CAD build for the part. Positions are in the model's coordinates, mm. Face numbers are marked on the shaded views. Coordinates: 2 decimals unless noted, no trailing zeros. Order: outer loops, then holes, each group sorted by start corner. A loop starts at its lowest first (then second) coordinate and runs counter-clockwise, first axis right, second up. Notation, with made-up numbers: M -9.75,-10.5 L 46.25,-10.5 A30 ccw 46.25,20.5 Z; hole C 74,-32.5 d10. An arc over 180 degrees is marked long. Write item = value, one per line.
from build123d import *


with BuildPart() as f1:
    # F0 (on Front) → F1 (revolve)
    with BuildSketch(Plane.XZ):
        Polygon((-22, 0), (-17, 0), (-16.25, 45), (-20.25, 45), align=None)
    revolve(axis=Axis((0, 0, 22.5), (0, 0, 1)))

    # F0 (on Front) → F2 (revolve)
    with BuildSketch(Plane.XZ):
        with BuildLine():
            Line((-20.25, 45), (-16.25, 45))
            Line((-16.25, 45), (-10.1249999976, 59.999902775))
            add(Edge.make_bspline(
                [(-10.1249999976, 59.999902775), (-8.5298389727, 64.666048141), (-6.5813622983, 69.2951174162), (-5.4999999953, 74.9998055501)],
                knots=[0, 0, 0, 0, 0.441861733, 0.441861733, 0.441861733, 0.441861733], degree=3))
            Line((-5.4999999953, 74.9998055501), (-8.4969373337, 75.1353289405))
            add(Edge.make_bspline(
                [(-14.1249999976, 59.999902775), (-12.3183567805, 64.7249967507), (-9.8064455142, 69.3661766921), (-8.4969373337, 75.1353289405)],
                knots=[0, 0, 0, 0, 0.4460290714, 0.4460290714, 0.4460290714, 0.4460290714], degree=3))
            Line((-14.1249999976, 59.999902775), (-20.25, 45))
        make_face()
    revolve(axis=Axis((0, 0, 60), (0, 0, 1)))

    # F0 (on Front) → F3 (revolve)
    with BuildSketch(Plane.XZ):
        with BuildLine():
            Line((-8.4969373337, 75.1353289405), (-5.4999999953, 74.9998055501))
            add(Edge.make_bspline(
                [(-5.4999999953, 74.9998055501), (-4.1340756876, 82.2056903566), (-4.1516769819, 91.1277804046), (-3.9999999953, 99.9998055501)],
                knots=[0.441861733, 0.441861733, 0.441861733, 0.441861733, 1, 1, 1, 1], degree=3))
            Line((-3.9999999953, 99.9998055501), (-3.9999999953, 124.9998055501))
            Line((-3.9999999953, 124.9998055501), (-6.9999999953, 124.9998055501))
            Line((-6.9999999953, 124.9998055501), (-6.9999999953, 99.9998055501))
            add(Edge.make_bspline(
                [(-8.4969373337, 75.1353289405), (-6.8705198887, 82.3006525327), (-7.0989050536, 91.2059633256), (-6.9999999953, 99.9998055501)],
                knots=[0.4460290714, 0.4460290714, 0.4460290714, 0.4460290714, 1, 1, 1, 1], degree=3))
        make_face()
    revolve(axis=Axis((0, 0, 100), (0, 0, 1)))


solid = f1.part
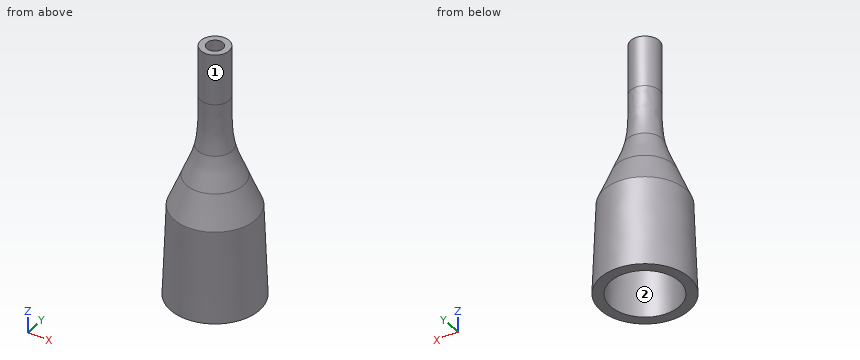
(1) Slice it at A-A, the plane z = 25.5. Write the cut outline in (x, y) (3 decimals).
Evaluation:
outline = C 0,0 d42.017; hole C 0,0 d33.15
(2) Wall check: line 1 (Y direction, x = 0, z = 116); line 2 (Y direction, x = 15, z = 5.5). Give the ranges that are in metal, low to high. Write a range as from..to.
Evaluation:
line_1 = -7..-4, 4..7
line_2 = -15.8..-7.8, 7.8..15.8
(3) Pin check, flat tips, straight feed: pin 1 Ø13 at (x, y) = (0, 0) entering from +Z; pin 2 Ø4 at (y, z) = (6, 105) entering from +X; pin 3 Ø10 at (x, z) = (11.5, 52) entering from +Y; pin 4 Ø6 at (x, z) = (-4, 62) entering from -Y. Stop position of each tip, or through.
Evaluation:
pin_1 = 125
pin_2 = 5.74
pin_3 = 17.07
pin_4 = -14.16
(4) Pull direction X, two halves, no side cores. Call the marked faces 1 and 2: +X half, -X half, draft (parallel to the pull), parting line (faces both ways), or undercut.
Evaluation:
face_1 = parting line
face_2 = undercut
(5) Slice it at B-B, the plane z = 53. Write the cut outline in (x, y).
Evaluation:
outline = C 0,0 d33.97; hole C 0,0 d25.97
